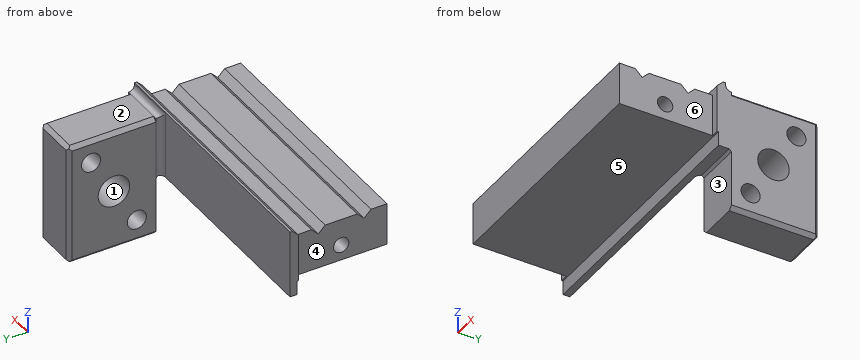
Autodesk Inventor part; units mm, degrees
ref_plane "HUB_XY" through (-6, 0, 0) normal (1, 0, 0) x (0, 0, -1)
ref_plane "HUB_YZ" through (-6, 0, 0) normal (0, 0, -1) x (0, 1, 0)
ref_plane "HUB_ZX" through (-6, 0, 0) normal (0, 1, 0) x (1, 0, 0)
sketch "Sketch_1" plane through (0, 0, 0) normal (1, 0, 0) x (0, 1, 0)
  line L0 (-12.3, 9) -> (-12.6, 9)
  line L1 (-12.6, 9) -> (-13.4, 8.2)
  line L2 (-13.4, 8.2) -> (-13.4, 7.5)
  line L3 (-13.4, 7.5) -> (-25.6, 7.5)
  line L4 (-25.6, 7.5) -> (-25.6, 1.95)
  line L5 (-25.6, 1.95) -> (-13.2, 1.95)
  line L6 (-13.2, 1.95) -> (-13.2, 0.1)
  line L7 (-13.2, 0.1) -> (-11.8, 0.1)
  line L8 (-11.8, 0.1) -> (-11.5, -0.2)
  line L9 (-11.5, -0.2) -> (-11.5, -8)
  line L10 (-11.5, -8) -> (-0.5, -8)
  line L11 (-0.5, -8) -> (0, -7.5)
  line L12 (0, -7.5) -> (0, 7.5)
  line L13 (0, 7.5) -> (-0.5, 8)
  line L14 (-0.5, 8) -> (-11.5, 8)
  arc A0 (-12.3, 8.8) -> (-11.5, 8) centre (-11.5, 8.8) ccw
  line L15 (-12.3, 8.8) -> (-12.3, 9)
extrude "Extrusion1" add sketch "Sketch_1" against normal blind 34
sketch "Sketch_2" plane through (0, 0, 0) normal (0, 0, 1) x (1, 0, 0)
  line L0 (-35, 1) -> (-35, -26.6)
  line L1 (-35, -26.6) -> (0, -26.6)
  line L2 (0, -26.6) -> (0, -13.4)
  line L3 (0, -13.4) -> (-1, -13.4)
  line L4 (-1, -13.4) -> (-1, -25.6)
  line L5 (-1, -25.6) -> (-33, -25.6)
  line L6 (-33, -25.6) -> (-33, -13.4)
  line L7 (-33, -13.4) -> (-34, -13.4)
  line L8 (-34, -13.4) -> (-34, -12.3)
  line L9 (-34, -12.3) -> (-6.8, -12.3)
  arc A0 (-6.8, -12.3) -> (-6, -11.5) centre (-6.8, -11.5) ccw
  line L10 (-6, -11.5) -> (-6, -0.5)
  line L11 (-6, -0.5) -> (-5.5, 0)
  line L12 (-5.5, 0) -> (-0.5, 0)
  line L13 (-0.5, 0) -> (0, -0.5)
  line L14 (0, -0.5) -> (0, 1)
  line L15 (0, 1) -> (-35, 1)
extrude "Extrusion2" cut sketch "Sketch_2" along normal mid plane 68
sketch "Sketch_3" plane through (0, 0, 0) normal (0, 1, 0) x (-1, 0, 0)
  circle A0 centre (0, 0) radius 34
  line L0 (6, -7.5) -> (6, 7.5)
  line L1 (6, 7.5) -> (5.5, 8)
  line L2 (5.5, 8) -> (0.5, 8)
  line L3 (0.5, 8) -> (0, 7.5)
  line L4 (0, 7.5) -> (0, -7.5)
  line L5 (0, -7.5) -> (0.5, -8)
  line L6 (0.5, -8) -> (5.5, -8)
  line L7 (5.5, -8) -> (6, -7.5)
extrude "Extrusion3" cut sketch "Sketch_3" against normal blind 11.5
sketch "Sketch_4" plane through (0, 0, 0) normal (1, 0, 0) x (0, 1, 0)
  line L0 (-14.7, 8.5) -> (-24.5, 8.5)
  line L1 (-24.5, 8.5) -> (-22.6, 6.6)
  line L2 (-22.6, 6.6) -> (-21.7, 7.5)
  line L3 (-21.7, 7.5) -> (-17.5, 7.5)
  line L4 (-17.5, 7.5) -> (-16.6, 6.6)
  line L5 (-16.6, 6.6) -> (-14.7, 8.5)
extrude "Extrusion4" cut sketch "Sketch_4" against normal blind 34
sketch "Sketch5" plane through (-6, -11.5, 7.5) normal (-1, 0, 0) x (0, 0, 1)
  point P0 (-7.5, 5.5)
hole "Hole1" at (-6, -6, 0) direction (1, 0, 0) diameter 4.134 depth 6
sketch "Sketch6" plane through (0, 0, 0) normal (1, 0, 0) x (0, 0, -1)
  point P0 (-5, -3)
hole "Hole2" at (0, -3, 5) direction (-1, 0, 0) diameter 2.5 depth 6
pattern_linear "Rectangular Pattern1" count 2 spacing 11.6619 along (0, -0.5145, -0.8575) of "Hole2"
sketch "Sketch7" plane through (-1, -25.6, 1.95) normal (1, 0, 0) x (0, 0, -1)
  point P0 (-2.05, 6)
hole "Hole3" at (-1, -19.6, 4) direction (-1, 0, 0) diameter 2.013 depth 7.5 tip angle 121
sketch "Sketch8" plane through (-33, -25.6, 1.95) normal (-1, 0, 0) x (0, 0, 1)
  point P0 (2.05, 6)
hole "Hole4" at (-33, -19.6, 4) direction (1, 0, 0) diameter 2.013 depth 7.5 tip angle 121
ref_plane "HUB_XY" through (-6, 0, 0) normal (1, 0, 0) x (0, 0, -1)
ref_plane "HUB_YZ" through (-6, 0, 0) normal (0, 0, -1) x (0, 1, 0)
ref_plane "HUB_ZX" through (-6, 0, 0) normal (0, 1, 0) x (1, 0, 0)
ref_plane "hal_1_XY" through (-1, -19.6, 4) normal (1, 0, 0) x (0, 0, -1)
ref_plane "hal_1_YZ" through (-1, -19.6, 4) normal (0, 0, -1) x (0, 1, 0)
ref_plane "hal_1_ZX" through (-1, -19.6, 4) normal (0, 1, 0) x (1, 0, 0)
ref_plane "hal_2_XY" through (-33, -19.6, 4) normal (1, 0, 0) x (0, 0, -1)
ref_plane "hal_2_YZ" through (-33, -19.6, 4) normal (0, 0, -1) x (0, 1, 0)
ref_plane "hal_2_ZX" through (-33, -19.6, 4) normal (0, 1, 0) x (1, 0, 0)
properties part number "SCHUNK-5521119 Finger EGP 40"
Input: part model. Units: mm. Frame: model coordinates. Face numbers are marked on the shaded views. A direction names the side the tool comes from. Give positions to 0.01 mm unless a question says otherwise; leave off trailing zeros. Order: outer loops, then holes, each group sorted by start corner. A loop starts at its lowest first (then second) coordinate and runs counter-clockwise, first axis right, second up.
Q1. Ray query, probe 1 along Z at (x, y) = (-2.5, -3); probe 2 along Z at (x, y) = (-5.25, -19.6); probe 3 along Y at (x, z) = (-26, 6.75). Return the intervals inside material, ascending.
Checked values:
probe 1: z = -8 to 3.75, 6.25 to 8
probe 2: z = 1.95 to 2.99, 5.01 to 7.5
probe 3: y = -25.6 to -22.75, -22.45 to -16.75, -16.45 to -12.3
Q2. Section C-C on x = -11.5. Output: boundary loops of the cut face in (y, z), and give its area (3 significant figures).
Checked values:
outline: (-25.6, 1.95) - (-13.2, 1.95) - (-13.2, 0.1) - (-12.3, 0.1) - (-12.3, 9) - (-12.6, 9) - (-13.4, 8.2) - (-13.4, 7.5) - (-15.7, 7.5) - (-16.6, 6.6) - (-17.5, 7.5) - (-21.7, 7.5) - (-22.6, 6.6) - (-23.5, 7.5) - (-25.6, 7.5) - close
area: 75.2 mm2
Q3. Set-up query: the marked faces 4, 5 and 6. Return all of +Z, -Z, +X, -X, +Y, -Y with unobstructed straight access to the full face (end or side cutting, diameter ignored); none if empty.
Checked values:
face 4: +Z, -Z, -X, -Y
face 5: -Z, +X, -X, -Y
face 6: +Z, -Z, +X, -Y
Q4. Contact query for flat-ended pins moving along their axis: pin 1 Ø10 at (x, y) = (-11, -20) entering from -Z; pin 2 Ø1.7 at (y, z) = (-20.5, 4) entering from -X; pin 3 Ø2.5 at (x, y) = (-13.5, -24.5) entering from +Z; pin 4 Ø3.5 at (y, z) = (-6, 0) entering from +X. Output: stop coordinate, or through.
Checked values:
pin 1: stops at z = 1.95
pin 2: stops at x = -33
pin 3: stops at z = 7.5
pin 4: passes through
Q5. Section B-B on z = -5. Output: boundary loops of the cut face in (x, y).
Checked values:
outline: (-6, -11.5) - (0, -11.5) - (0, -10.25) - (-6, -10.25) - close; (-6, -7.75) - (0, -7.75) - (0, -0.5) - (-0.5, 0) - (-5.5, 0) - (-6, -0.5) - close
Q6. Section D-D on y = -3. Output: boundary loops of the cut face in (x, z).
Checked values:
outline: (-6, -7.5) - (-5.5, -8) - (-0.5, -8) - (0, -7.5) - (0, 3.75) - (-6, 3.75) - close; (-6, 6.25) - (0, 6.25) - (0, 7.5) - (-0.5, 8) - (-5.5, 8) - (-6, 7.5) - close
Q7. Draft query along Z for the marked faces 1, 2 and 3. Return one class per face: +Z half, -Z half, draft (parallel to the pull), parting line (faces both ways), or undercut.
Checked values:
face 1: undercut
face 2: +Z half
face 3: draft
Q8. Section A-A on y = -6. Output: boundary loops of the cut face in (x, z).
Checked values:
outline: (-6, -7.5) - (-5.5, -8) - (-0.5, -8) - (0, -7.5) - (0, -2.07) - (-6, -2.07) - close; (-6, 2.07) - (0, 2.07) - (0, 7.5) - (-0.5, 8) - (-5.5, 8) - (-6, 7.5) - close
